Study the drawing (mm; zero at the part's minimum x, y, z) and answer. A direction names the side the tool comes from. Round coordinates to 2 decimals unless told otherwise and drop trailing zeros. Write each loop counter-clockwise with the first axis right and the second up, starting at its lowest first coordinate (ties: lowest second). Pieces come first, ordered by that corner, then holes.
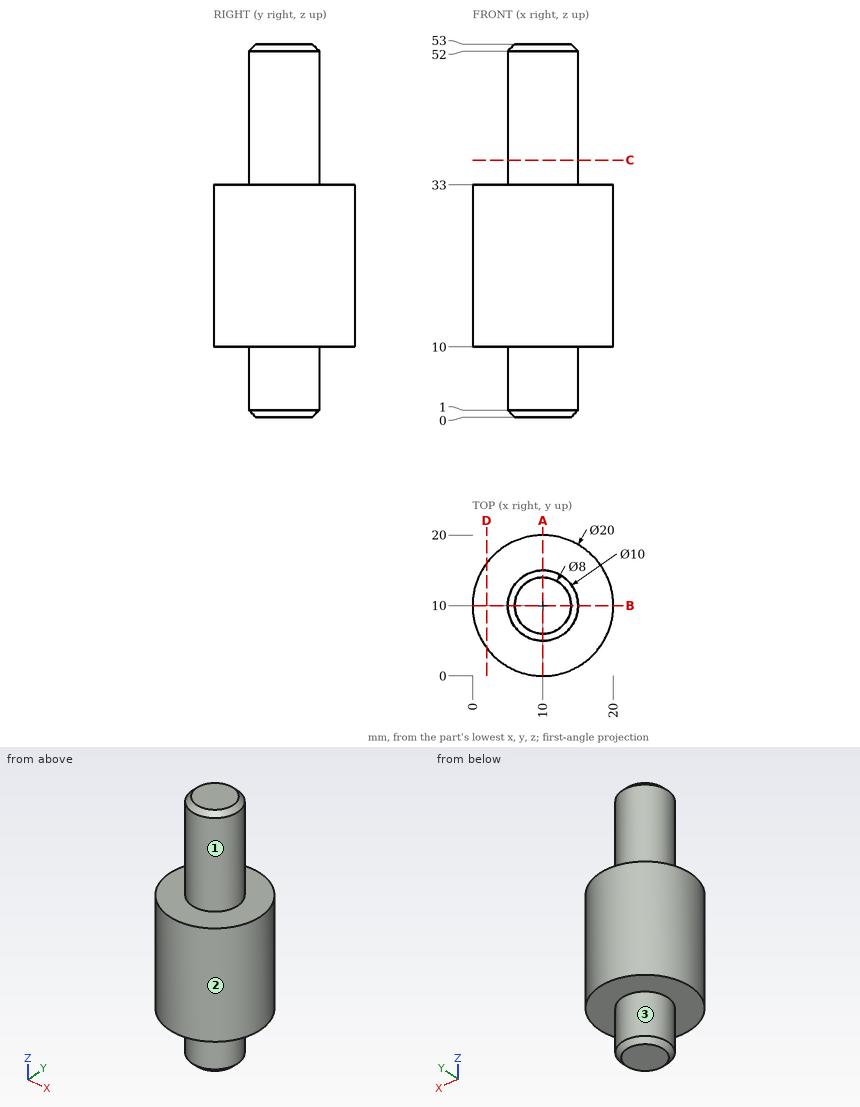
Q1. Find section A-A (x = 10). Determine the outline of the cut face in (y, z), plus the area to 3 significant figures.
Q2. Given pin 1 (8 mm diameter, centred on x = 18, z = 16, fed in from -Y); pin 2 (2 mm diameter, centred on x = 15.5, y = 16.5, fed in from -Z); pin 3 (4 mm diameter, centred on y = 17, z = 16.5, fed in from -X), each flat-ended and moving along its own axis, determine where each tip first touches the part or whether it passes through.
Q3. Find section D-D (x = 2). Determine the outline of the cut face in (y, z).
Q4. Find section C-C (z = 36.5). Determine the outline of the cut face in (x, y), plus the area to 3 significant figures.
Q5. A tool of negligible diameter and unlimited length cuts with its end or side. For the marked faces 1, 2 and 3, from which of +Z, -Z, +X, -X, +Y, -Y can it reach the whole face along a straight path? Write none if from no direction.
Q6. Find the intervals of material crossed by L1, parallel to Z at x = 3.75, y = 15.5; L2, parallel to X at y = 10.25, z = 6; L3, parallel to X at y = 12.75, z = 42, in increasing order.
Report:
1. outline: (0, 10) - (5, 10) - (5, 1) - (6, 0) - (14, 0) - (15, 1) - (15, 10) - (20, 10) - (20, 33) - (15, 33) - (15, 52) - (14, 53) - (6, 53) - (5, 52) - (5, 33) - (0, 33) - close
1. area: 758 mm2
2. pin 1: stops at y = 0.83
2. pin 2: stops at z = 10
2. pin 3: stops at x = 1.34
3. outline: (4, 10) - (16, 10) - (16, 33) - (4, 33) - close
4. outline: circle Ø10 at (10, 10)
4. area: 78.5 mm2
5. face 1: +Z
5. face 2: +Z, -Z
5. face 3: -Z
6. L1: z = 10 to 33
6. L2: x = 5.01 to 14.99
6. L3: x = 5.82 to 14.18
